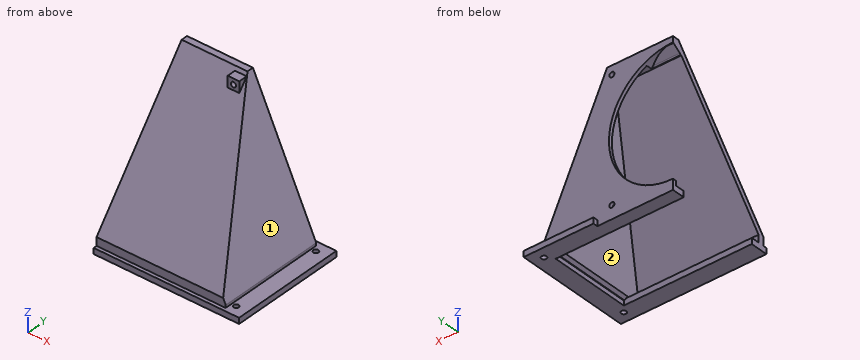
from build123d import *

# Parameters (mm, degrees)
BOX015_W               = 30
BOX015_H               = 9
BOX015_DEPTH           = 5
BOX015_ROLL_ANGLE      = 36
CHAMFER005_SIZE        = 1
BOX014_W               = 150
BOX014_H               = 150
BOX014_DEPTH           = 150
CYLINDER007_R          = 2.2
CYLINDER007_DEPTH      = 50
CYLINDER005_R          = 2.2
CYLINDER005_DEPTH      = 50
CYLINDER006_R          = 2.2
CYLINDER006_DEPTH      = 50
CYLINDER004_R          = 2.2
CYLINDER004_DEPTH      = 50
FUSION_ROLL_ANGLE      = -90
BOX013_W               = 10
BOX013_H               = 8
BOX013_DEPTH           = 10
CHAMFER003_SIZE        = 6
BOX012_W               = 10
BOX012_H               = 8
BOX012_DEPTH           = 10
CHAMFER002_SIZE        = 6
BOX011_W               = 130
BOX011_H               = 10
BOX011_DEPTH           = 10
CYLINDER002_R          = 2.2
CYLINDER002_DEPTH      = 50
CYLINDER003_R          = 2.2
CYLINDER003_DEPTH      = 50
CYLINDER001_R          = 2.2
CYLINDER001_DEPTH      = 50
CYLINDER_R             = 2.2
CYLINDER_DEPTH         = 50
BOX001_W               = 220
BOX001_H               = 70
BOX001_DEPTH           = 12
BOX_W                  = 250
BOX_H                  = 100
BOX_DEPTH              = 5
CYLINDER008_R          = 55
CYLINDER008_DEPTH      = 10
CYLINDER008_ROLL_ANGLE = 90
BOX010_W               = 300
BOX010_H               = 20
BOX010_DEPTH           = 41
BOX008_W               = 234
BOX008_H               = 93
BOX008_DEPTH           = 249
BOX008_ROLL_ANGLE      = -38
BOX009_W               = 120
BOX009_H               = 104
BOX009_DEPTH           = 200
BOX009_PLACEMENT_ANGLE = 25
BOX006_W               = 120
BOX006_H               = 104
BOX006_DEPTH           = 200
BOX006_PLACEMENT_ANGLE = 25
BOX007_W               = 222
BOX007_H               = 93
BOX007_DEPTH           = 120
BOX004_W               = 234
BOX004_H               = 93
BOX004_DEPTH           = 249
BOX004_ROLL_ANGLE      = -38
BOX005_W               = 120
BOX005_H               = 104
BOX005_DEPTH           = 200
BOX005_PLACEMENT_ANGLE = 25
BOX002_W               = 120
BOX002_H               = 104
BOX002_DEPTH           = 200
BOX002_PLACEMENT_ANGLE = 25
BOX003_W               = 222
BOX003_H               = 93
BOX003_DEPTH           = 120
CHAMFER_SIZE           = 2
CHAMFER001_SIZE        = 2
CHAMFER004_SIZE        = 1


with BuildPart() as chamfer005:
    # Box015 → Box015 (new body)
    with BuildSketch(Plane.XY):
        with Locations((15, 4.5)):
            Rectangle(BOX015_W, BOX015_H)
    extrude(amount=BOX015_DEPTH)


with BuildPart() as chamfer005_1:
    # Box015 roll: moved
    add(chamfer005.part.rotate(Axis((0, 0, 0), (1, 0, 0)), BOX015_ROLL_ANGLE))


with BuildPart() as chamfer005_2:
    # Box015 placement: moved
    add(chamfer005_1.part.moved(Location((-30, 39, 114))))

    # Chamfer005
    chamfer005_edges = [chamfer005_2.edges().sort_by_distance(p)[0] for p in [
        (-15, 46.281153, 119.290067),
    ]]
    chamfer(chamfer005_edges, length=CHAMFER005_SIZE)


with BuildPart() as cube014:
    # Box014 → Box014 (new body)
    with BuildSketch(Plane(origin=(0, -70, -1), x_dir=(1, 0, 0), z_dir=(0, 0, 1))):
        with Locations((75, 75)):
            Rectangle(BOX014_W, BOX014_H)
    extrude(amount=BOX014_DEPTH)


with BuildPart() as cylinder007:
    # Cylinder007 → Cylinder007 (new body)
    with BuildSketch(Plane(origin=(52.5, -52.5, 0), x_dir=(1, 0, 0), z_dir=(0, 0, 1))):
        Circle(CYLINDER007_R)
    extrude(amount=CYLINDER007_DEPTH)


with BuildPart() as cylinder005:
    # Cylinder005 → Cylinder005 (new body)
    with BuildSketch(Plane(origin=(52.5, 52.5, 0), x_dir=(1, 0, 0), z_dir=(0, 0, 1))):
        Circle(CYLINDER005_R)
    extrude(amount=CYLINDER005_DEPTH)


with BuildPart() as cylinder006:
    # Cylinder006 → Cylinder006 (new body)
    with BuildSketch(Plane(origin=(-52.5, 52.5, 0), x_dir=(1, 0, 0), z_dir=(0, 0, 1))):
        Circle(CYLINDER006_R)
    extrude(amount=CYLINDER006_DEPTH)


with BuildPart() as fan_holes:
    # Cylinder004 → Cylinder004 (new body)
    with BuildSketch(Plane(origin=(-52.5, -52.5, 0), x_dir=(1, 0, 0), z_dir=(0, 0, 1))):
        Circle(CYLINDER004_R)
    extrude(amount=CYLINDER004_DEPTH)

    # Fusion: union Cylinder007, Cylinder005, Cylinder006
    add(cylinder007.part)
    add(cylinder005.part)
    add(cylinder006.part)


with BuildPart() as fan_holes_1:
    # Fusion roll: moved
    add(fan_holes.part.rotate(Axis((0, 0, 0), (1, 0, 0)), FUSION_ROLL_ANGLE))


with BuildPart() as fan_holes_2:
    # Fusion placement: moved
    add(fan_holes_1.part.moved(Location((0, 15, 64))))


with BuildPart() as chamfer003:
    # Box013 → Box013 (new body)
    with BuildSketch(Plane(origin=(47.5, 31, 111.5), x_dir=(1, 0, 0), z_dir=(0, 0, 1))):
        with Locations((5, 4)):
            Rectangle(BOX013_W, BOX013_H)
    extrude(amount=BOX013_DEPTH)

    # Chamfer003
    chamfer003_edges = [chamfer003.edges().sort_by_distance(p)[0] for p in [
        (52.5, 39, 111.5),
    ]]
    chamfer(chamfer003_edges, length=CHAMFER003_SIZE)


with BuildPart() as part_mirroring002:
    # Part__Mirroring002: instance of Chamfer003
    add(chamfer003.part.mirror(Plane(origin=(0, 0, 0), x_dir=(0, -1, 0), z_dir=(1, 0, 0))))


with BuildPart() as chamfer002:
    # Box012 → Box012 (new body)
    with BuildSketch(Plane(origin=(47.5, 31, 111.5), x_dir=(1, 0, 0), z_dir=(0, 0, 1))):
        with Locations((5, 4)):
            Rectangle(BOX012_W, BOX012_H)
    extrude(amount=BOX012_DEPTH)

    # Chamfer002
    chamfer002_edges = [chamfer002.edges().sort_by_distance(p)[0] for p in [
        (52.5, 39, 111.5),
    ]]
    chamfer(chamfer002_edges, length=CHAMFER002_SIZE)


with BuildPart() as cube011:
    # Box011 → Box011 (new body)
    with BuildSketch(Plane(origin=(-65, 46, -2), x_dir=(1, 0, 0), z_dir=(0, 0, 1))):
        with Locations((65, 5)):
            Rectangle(BOX011_W, BOX011_H)
    extrude(amount=BOX011_DEPTH)


with BuildPart() as cylinder002:
    # Cylinder002 → Cylinder002 (new body)
    with BuildSketch(Plane(origin=(-115, 41, 0), x_dir=(1, 0, 0), z_dir=(0, 0, 1))):
        Circle(CYLINDER002_R)
    extrude(amount=CYLINDER002_DEPTH)


with BuildPart() as cylinder003:
    # Cylinder003 → Cylinder003 (new body)
    with BuildSketch(Plane(origin=(115, 41, 0), x_dir=(1, 0, 0), z_dir=(0, 0, 1))):
        Circle(CYLINDER003_R)
    extrude(amount=CYLINDER003_DEPTH)


with BuildPart() as cylinder001:
    # Cylinder001 → Cylinder001 (new body)
    with BuildSketch(Plane(origin=(115, -41, 0), x_dir=(1, 0, 0), z_dir=(0, 0, 1))):
        Circle(CYLINDER001_R)
    extrude(amount=CYLINDER001_DEPTH)


with BuildPart() as mount_holes:
    # Cylinder → Cylinder (new body)
    with BuildSketch(Plane(origin=(-115, -41, 0), x_dir=(1, 0, 0), z_dir=(0, 0, 1))):
        Circle(CYLINDER_R)
    extrude(amount=CYLINDER_DEPTH)

    # Fusion001: union Cylinder002, Cylinder003, Cylinder001
    add(cylinder002.part)
    add(cylinder003.part)
    add(cylinder001.part)


with BuildPart() as mount_holes_1:
    # Fusion001 placement: moved
    add(mount_holes.part.moved(Location((0, 0, -1))))


with BuildPart() as cube001:
    # Box001 → Box001 (new body)
    with BuildSketch(Plane(origin=(-110, -35, -1), x_dir=(1, 0, 0), z_dir=(0, 0, 1))):
        with Locations((110, 35)):
            Rectangle(BOX001_W, BOX001_H)
    extrude(amount=BOX001_DEPTH)


with BuildPart() as cut001:
    # Box → Box (new body)
    with BuildSketch(Plane(origin=(-125, -50, 0), x_dir=(1, 0, 0), z_dir=(0, 0, 1))):
        with Locations((125, 50)):
            Rectangle(BOX_W, BOX_H)
    extrude(amount=BOX_DEPTH)

    # Cut: cut Cube001
    add(cube001.part, mode=Mode.SUBTRACT)

    # Cut001: cut mount-holes
    add(mount_holes_1.part, mode=Mode.SUBTRACT)


with BuildPart() as cylinder008:
    # Cylinder008 → Cylinder008 (new body)
    with BuildSketch(Plane.XY):
        Circle(CYLINDER008_R)
    extrude(amount=CYLINDER008_DEPTH)


with BuildPart() as cylinder008_1:
    # Cylinder008 roll: moved
    add(cylinder008.part.rotate(Axis((0, 0, 0), (1, 0, 0)), CYLINDER008_ROLL_ANGLE))


with BuildPart() as cylinder008_2:
    # Cylinder008 placement: moved
    add(cylinder008_1.part.moved(Location((0, 49, 64))))


with BuildPart() as cube010:
    # Box010 → Box010 (new body)
    with BuildSketch(Plane(origin=(-150, -62, -12), x_dir=(1, 0, 0), z_dir=(0, 0, 1))):
        with Locations((150, 10)):
            Rectangle(BOX010_W, BOX010_H)
    extrude(amount=BOX010_DEPTH)


with BuildPart() as cube008:
    # Box008 → Box008 (new body)
    with BuildSketch(Plane.XY):
        with Locations((117, 46.5)):
            Rectangle(BOX008_W, BOX008_H)
    extrude(amount=BOX008_DEPTH)


with BuildPart() as cube008_1:
    # Box008 roll: moved
    add(cube008.part.rotate(Axis((0, 0, 0), (1, 0, 0)), BOX008_ROLL_ANGLE))


with BuildPart() as cube008_2:
    # Box008 placement: moved
    add(cube008_1.part.moved(Location((-121, -144, 39))))


with BuildPart() as cube009:
    # Box009 → Box009 (new body)
    with BuildSketch(Plane.XY):
        with Locations((60, 52)):
            Rectangle(BOX009_W, BOX009_H)
    extrude(amount=BOX009_DEPTH)


with BuildPart() as cube009_1:
    # Box009 placement: moved
    add(cube009.part.moved(Location((-245, -55, 4))).rotate(Axis((-245, -55, 4), (0, 1, 0)), BOX009_PLACEMENT_ANGLE))


with BuildPart() as part_mirroring001:
    # Part__Mirroring001: instance of Cube009
    add(cube009_1.part.mirror(Plane(origin=(0, 0, 0), x_dir=(0, -1, 0), z_dir=(1, 0, 0))))


with BuildPart() as fusion003:
    # Box006 → Box006 (new body)
    with BuildSketch(Plane.XY):
        with Locations((60, 52)):
            Rectangle(BOX006_W, BOX006_H)
    extrude(amount=BOX006_DEPTH)


with BuildPart() as fusion003_1:
    # Box006 placement: moved
    add(fusion003.part.moved(Location((-245, -55, 4))).rotate(Axis((-245, -55, 4), (0, 1, 0)), BOX006_PLACEMENT_ANGLE))

    # Fusion003: union Part__Mirroring001
    add(part_mirroring001.part)


with BuildPart() as cut006:
    # Box007 → Box007 (new body)
    with BuildSketch(Plane(origin=(-111, -47, 4), x_dir=(1, 0, 0), z_dir=(0, 0, 1))):
        with Locations((111, 46.5)):
            Rectangle(BOX007_W, BOX007_H)
    extrude(amount=BOX007_DEPTH)

    # Cut004: cut Fusion003
    add(fusion003_1.part, mode=Mode.SUBTRACT)

    # Cut005: cut Cube008
    add(cube008_2.part, mode=Mode.SUBTRACT)


with BuildPart() as cut006_1:
    # Cut005 placement: moved
    add(cut006.part.moved(Location((0, -3, -11))))

    # Cut006: cut Cube010
    add(cube010.part, mode=Mode.SUBTRACT)


with BuildPart() as cube004:
    # Box004 → Box004 (new body)
    with BuildSketch(Plane.XY):
        with Locations((117, 46.5)):
            Rectangle(BOX004_W, BOX004_H)
    extrude(amount=BOX004_DEPTH)


with BuildPart() as cube004_1:
    # Box004 roll: moved
    add(cube004.part.rotate(Axis((0, 0, 0), (1, 0, 0)), BOX004_ROLL_ANGLE))


with BuildPart() as cube004_2:
    # Box004 placement: moved
    add(cube004_1.part.moved(Location((-121, -144, 39))))


with BuildPart() as cube005:
    # Box005 → Box005 (new body)
    with BuildSketch(Plane.XY):
        with Locations((60, 52)):
            Rectangle(BOX005_W, BOX005_H)
    extrude(amount=BOX005_DEPTH)


with BuildPart() as cube005_1:
    # Box005 placement: moved
    add(cube005.part.moved(Location((-245, -55, 4))).rotate(Axis((-245, -55, 4), (0, 1, 0)), BOX005_PLACEMENT_ANGLE))


with BuildPart() as part_mirroring:
    # Part__Mirroring: instance of Cube005
    add(cube005_1.part.mirror(Plane(origin=(0, 0, 0), x_dir=(0, -1, 0), z_dir=(1, 0, 0))))


with BuildPart() as fusion002:
    # Box002 → Box002 (new body)
    with BuildSketch(Plane.XY):
        with Locations((60, 52)):
            Rectangle(BOX002_W, BOX002_H)
    extrude(amount=BOX002_DEPTH)


with BuildPart() as fusion002_1:
    # Box002 placement: moved
    add(fusion002.part.moved(Location((-245, -55, 4))).rotate(Axis((-245, -55, 4), (0, 1, 0)), BOX002_PLACEMENT_ANGLE))

    # Fusion002: union Part__Mirroring
    add(part_mirroring.part)


with BuildPart() as fusion006:
    # Box003 → Box003 (new body)
    with BuildSketch(Plane(origin=(-111, -47, 4), x_dir=(1, 0, 0), z_dir=(0, 0, 1))):
        with Locations((111, 46.5)):
            Rectangle(BOX003_W, BOX003_H)
    extrude(amount=BOX003_DEPTH)

    # Cut002: cut Fusion002
    add(fusion002_1.part, mode=Mode.SUBTRACT)

    # Cut003: cut Cube004
    add(cube004_2.part, mode=Mode.SUBTRACT)

    # Cut007: cut Cut006
    add(cut006_1.part, mode=Mode.SUBTRACT)

    # Cut008: cut Cylinder008
    add(cylinder008_2.part, mode=Mode.SUBTRACT)

    # Fusion004: union Cut001
    add(cut001.part)

    # Cut009: cut Cube011
    add(cube011.part, mode=Mode.SUBTRACT)

    # Chamfer
    chamfer_edges = [fusion006.edges().sort_by_distance(p)[0] for p in [
        (107.465265, 0, 4),
    ]]
    chamfer(chamfer_edges, length=CHAMFER_SIZE)

    # Chamfer001
    chamfer001_edges = [fusion006.edges().sort_by_distance(p)[0] for p in [
        (-107.465265, 0, 4),
    ]]
    chamfer(chamfer001_edges, length=CHAMFER001_SIZE)

    # Fusion005: union Part__Mirroring002, Chamfer002
    add(part_mirroring002.part)
    add(chamfer002.part)

    # Cut010: cut fan-holes
    add(fan_holes_2.part, mode=Mode.SUBTRACT)

    # Chamfer004
    chamfer004_edges = [fusion006.edges().sort_by_distance(p)[0] for p in [
        (0, 39, 113),
    ]]
    chamfer(chamfer004_edges, length=CHAMFER004_SIZE)

    # Cut011: cut Cube014
    add(cube014.part, mode=Mode.SUBTRACT)

    # Fusion006: union Chamfer005
    add(chamfer005_2.part)


with BuildPart() as part_mirroring003:
    # Part__Mirroring003: instance of Fusion006
    add(fusion006.part.mirror(Plane(origin=(0, 0, 0), x_dir=(0, -1, 0), z_dir=(1, 0, 0))))


solid = part_mirroring003.part
The model under review builds one solid part; all positions refer to its coordinate system, in mm. Face numbers are marked on the shaded views. Round coordinates to 2 decimals unless told otherwise and drop trailing zeros. Loops run counter-clockwise (first coordinate to the right, second up) from the corner with the lowest first, then second, coordinate; pieces in that order, holes last. Notation, with made-up numbers: (10.25, -35.5) - (15.25, -35.5) arc R24 ccw to (15.25, -0.5) - close; hole circle Ø7 at (77, -15.5). An arc over 180 degrees is marked (long way). Use CSV: the item, a comma, the result in double quotes.
(1) Clearance check with flat-ended pins moving along their axes: P1, Ø4, axis at x = 78, y = 40.5, coming from the +Z side; P2, Ø4, axis at x = 90.5, y = 3.5, coming from the -Z side; P3, Ø3.5, axis at x = 79, y = -37.5, coming from the +Z side. State where each tip first meets the part, or that it passes through.
Working result:
P1,"stops at z = 82.48"
P2,"stops at z = 36.09"
P3,"stops at z = 26.5"
(2) Take a section at C-C, the plane x = 52.5. State how many separate pieces and enclosed holes the cut face has, plus the area to 3 significant figures.
Working result:
separate pieces,"4"
enclosed holes,"0"
area,"1,020 mm^2"
(3) Take a section at D-D, the plane y = 19. Give the boundary of the cut face in (x, z), plus the area to 3 significant figures.
Working result:
outline,"(0, 89.41) - (67.64, 89.41) - (106.62, 5.81) - (109.47, 4) - (110, 4) - (110, 0) - (125, 0) - (125, 5) - (111, 5) - (111, 7.42) - (69.43, 96.57) - (0, 96.57) - close"
area,"1,020 mm^2"
(4) The part is to be moulded in two halves that separate along Y. For the marked faces 1 and 2, say which applies: pulls with the +Y half, pulls with the -Y half, needs draft (parallel to the pull), parting line crosses it, or undercut.
Working result:
face 1,"needs draft"
face 2,"undercut"
(5) For line 1 (Y direction, x = 115, z = 3); line 2 (Z direction, x = 52.5, y = 42); line 3 (X direction, y = 41, z = 1), list the stretches that pass through material, from the lowest coordinate up.
Working result:
line 1,"y = -50 to -43.2, -38.8 to 38.8, 43.2 to 50"
line 2,"z = 0 to 5, 113 to 114.3, 118.7 to 124"
line 3,"x = 0 to 112.8, 117.2 to 125"
(6) Take a section at B-B, the plane z = 57.5. Give the boundary of the cut face in (x, y).
Working result:
outline,"(0, -11.53) - (87.65, -11.53) - (87.65, 46) - (54.61, 46) - (54.61, 43) - (82.52, 43) - (82.52, -5.93) - (0, -5.93) - close"
(7) Take a section at A-A, the plane x = 17.5. Give the boundary of the cut face in (y, z).
Working result:
outline,"(-50, 0) - (-35, 0) - (-35, 5) - (-42, 5) - (-42, 11.34) - (37.43, 113) - (38, 113) - (39, 114) - (41.95, 116.14) - (46, 116.14) - (46, 124) - (40.43, 124) - (-47, 12.1) - (-47, 5) - (-50, 5) - close; (35, 0) - (46, 0) - (46, 11.86) - (43, 11.86) - (43, 5) - (35, 5) - close"
